Part model, mm, in its own coordinate system. Face numbers are marked on the shaded views. A direction names the side the tool comes from. Round coordinates to 2 decimals unless told otherwise and drop trailing zeros. Write each loop counter-clockwise with the first axis right and the second up, starting at its lowest first coordinate (ties: lowest second). Pieces come first, ordered by that corner, then holes.
```python
from build123d import *

# Parameters (mm, degrees)
F0_W     = 0.9875223041
F0_H     = 0.4511103034
F0_W_2   = 1.6117542982
F0_H_2   = 0.2151634544
F0_W_3   = 2.0527206361
F0_H_3   = 0.3410726786
F1_DEPTH = 25


with BuildPart() as f1:
    # F0 (on Front) → F1 (new body)
    with BuildSketch(Plane.XZ):
        Polygon((-5.0200670958, 17.5655037165), (-9.5167346299, 17.5655037165), (-9.5167346299, 15.2649758384), (-7.4343085289, 15.2649758384), (-7.4343085289, 11.3675463945), (-5.0200670958, 11.3675463945), align=None)
        Polygon((-9.5167346299, 23.2478547841), (-13.7016326189, 23.2478547841), (-13.7016326189, 11.4775840193), (-12.0863057673, 11.4775840193), (-12.0863057673, 15.2649758384), (-9.5167346299, 15.2649758384), (-9.5167346299, 17.5655037165), align=None)
        Polygon((-12.0863057673, 15.2649758384), (-12.0863057673, 11.4775840193), (-11.0987834632, 11.4775840193), (-11.0987834632, 12.3073123395), (-9.5167346299, 12.3073123395), (-9.5167346299, 15.2649758384), align=None)
        with Locations((-11.5925446153, 11.2520288676)):
            Rectangle(F0_W, F0_H)
        Polygon((-7.4343085289, 15.2649758384), (-9.5167346299, 15.2649758384), (-9.5167346299, 12.3073123395), (-9.487029165, 12.3073123395), (-9.487029165, 11.3675463945), (-7.4343085289, 11.3675463945), align=None)
        Polygon((-9.5167346299, 11.4775840193), (-11.0987834632, 11.4775840193), (-11.0987834632, 11.0264737159), (-9.487029165, 11.0264737159), (-9.487029165, 11.3675463945), (-9.5167346299, 11.3675463945), align=None)
        with Locations((-10.2929063141, 10.9188919887)):
            Rectangle(F0_W_2, F0_H_2)
        with Locations((-8.460668847, 11.1970100552)):
            Rectangle(F0_W_3, F0_H_3)
    extrude(amount=F1_DEPTH)


solid = f1.part
```
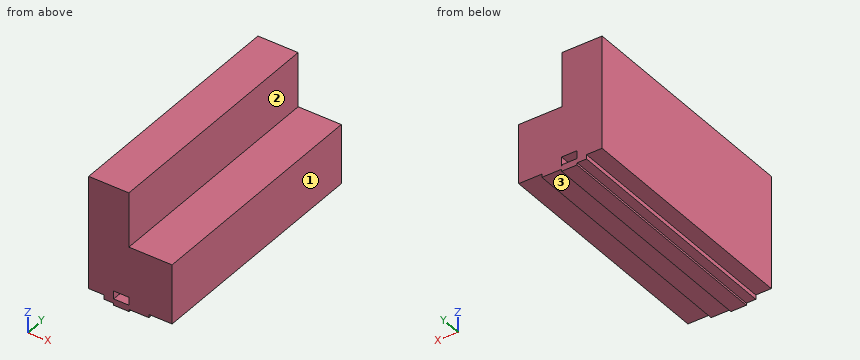
Q1. Cut at A-A on z = 12. Write the cut outline in (x, y), plus the area to 3 significant figures.
Values follow:
outline: (-13.7, -25) - (-11.1, -25) - (-11.1, 0) - (-13.7, 0) - close; (-9.49, -25) - (-5.02, -25) - (-5.02, 0) - (-9.49, 0) - close
area: 177 mm2
Q2. Wall check: L1, parallel to X at y = -5.25, z = 11.75; L2, parallel to Z at x = -9.75, y = -13.75; L3, parallel to Z at x = -5.5, y = -3.25. Give the ranges that are in metal, low to high.
Values follow:
L1: x = -13.7 to -11.1, -9.49 to -5.02
L2: z = 10.81 to 11.48, 12.31 to 23.25
L3: z = 11.37 to 17.57
Q3. Cut at B-B on x = -10. Write the cut outline in (y, z).
Values follow:
outline: (-25, 10.81) - (0, 10.81) - (0, 11.48) - (-25, 11.48) - close; (-25, 12.31) - (0, 12.31) - (0, 23.25) - (-25, 23.25) - close
Q4. Which spindle directions (+Z, -Z, +X, -X, +Y, -Y) get a long thin tool onto all of the face, cutting with end or side? Do the marked faces 1, 2 and 3. Say none if no direction does.
Values follow:
face 1: +Z, -Z, +X, +Y, -Y
face 2: +Z, +X, +Y, -Y
face 3: -Z, +X, +Y, -Y
Q5. Drop flat-ended pins along their axis: pin 1 (1.1 mm diameter, centred on x = -12, y = -18.5, fed in from -Z); pin 2 (2 mm diameter, centred on x = -7, y = -6.5, fed in from +Z); pin 3 (1.2 mm diameter, centred on x = -6, y = -14.5, fed in from -Z). Give the stop position or say it passes through.
Values follow:
pin 1: stops at z = 11.03
pin 2: stops at z = 17.57
pin 3: stops at z = 11.37
Q6. Cut at D-D on x = -7.75. Write the cut outline in (y, z).
Values follow:
outline: (-25, 11.03) - (0, 11.03) - (0, 17.57) - (-25, 17.57) - close
